from build123d import *

# Parameters (mm, degrees)
SKETCH1_W           = 12.7
SKETCH1_H           = 12.7
BOSS_EXTRUDE1_DEPTH = 2.54
FILLET1_R           = 0.635
SHELL1_START        = 0.635
SHELL1_OUTLINE_W    = 1.905
SHELL1_OUTLINE_H    = 11.43
SHELL1_DEPTH        = 11.43
SKETCH2_R           = 2.54
BOSS_EXTRUDE2_DEPTH = 1.905
BOSS_EXTRUDE3_DEPTH = 0.00254


# Read off the part's stored shape, not the designer's step: Shell1
with BuildPart() as part:
    # Sketch1 → Boss-Extrude1 (new body)
    with BuildSketch(Plane(origin=(0, 0, 0), x_dir=(1, 0, 0), z_dir=(0, 1, 0))):
        with Locations((6.35, 6.35)):
            Rectangle(SKETCH1_W, SKETCH1_H)
    extrude(amount=BOSS_EXTRUDE1_DEPTH)

    # Fillet1
    fillet1_edges = [part.edges().sort_by_distance(p)[0] for p in [
        (0, 1.27, -12.7),
        (12.7, 1.27, -12.7),
        (12.7, 1.27, 0),
        (0, 1.27, 0),
    ]]
    fillet(fillet1_edges, radius=FILLET1_R)

    # Shell1 outline → Shell1 (cut)
    with BuildSketch(Plane.YZ.offset(SHELL1_START)):
        with Locations((0.9525, -6.35)):
            Rectangle(SHELL1_OUTLINE_W, SHELL1_OUTLINE_H)
    extrude(amount=SHELL1_DEPTH, mode=Mode.SUBTRACT)

    # Sketch2 → Boss-Extrude2 (add)
    with BuildSketch(Plane(origin=(0, 1.905, 0), x_dir=(-1, 0, 0), z_dir=(0, -1, 0))):
        with Locations(Location((-6.35, 6.35, 0), (0, 0, 270))):
            Circle(SKETCH2_R)
    extrude(amount=BOSS_EXTRUDE2_DEPTH)

    # Sketch3 → Boss-Extrude3 (add)
    with BuildSketch(Plane(origin=(0, 2.54, 0), x_dir=(1, 0, 0), z_dir=(0, 1, 0))):
        Polygon((4.556857692, 8.001), (5.145173998, 8.001), (5.615191026, 5.974011819), (6.153897957, 8.001), (6.707869311, 8.001), (7.243396154, 5.974011819), (7.712141146, 8.001), (8.301729487, 8.001), (7.567129127, 4.826), (6.971816627, 4.826), (6.42929359, 6.878428886), (5.883590465, 4.826), (5.292730088, 4.826), align=None)
    extrude(amount=BOSS_EXTRUDE3_DEPTH)


solid = part.part
Design review of the part built by this model. Coordinates are the model's own, in mm. A direction names the side the tool comes from. Round coordinates to 2 decimals unless told otherwise and drop trailing zeros. Write each loop counter-clockwise with the first axis right and the second up, starting at its lowest first coordinate (ties: lowest second). Pieces come first, ordered by that corner, then holes. Notation, with made-up numbers: M -15,68.25 L 0,68.25 A13 ccw 0,84.25 Z; hole C 27,89.5 d7. An arc over 180 degrees is marked long. One line per item, written item: value. Start each with the question number.
1. Draft analysis for pull direction Z (two halves, no side actions). For faces 1 (the face through (6, 1, 0)), 2 (the face through (0.635, 1, -6)), 3 (the face through (0, 1, -6)), state which applies: pulls with the +Z half, pulls with the -Z half, needs draft (parallel to the pull), parting line crosses it, or undercut.
2. Take a section at C-C on z = -2.5. State the section outline as (x, y) points (3 decimals), then the cut area to 3 significant figures.
3. Take a section at D-D on z = -8.5. State the section outline as (x, y) points (3 decimals), then the cut area to 3 significant figures.
4. Clearance check with a flat-ended pin moving along its axis: P1, Ø1.5, axis at x = 8, z = -5.5, coming from the +Y side. State where the tip first meets the part, or that it passes through.
5. Take a section at B-B on x = 10.75. State the section outline as (y, z) points (3 decimals).
6. Take a section at A-A on y = 1.7. State the section outline as (x, z) points (3 decimals).
7. To check wall thickness, follow probe 1 along X at (y, z) = (1.5, -6.25) (3 decimals); probe 2 along X at (y, z) = (0.4, -10.25) (3 decimals); probe 3 along Z at (x, y) = (11.5, 0.7) (3 decimals). State the ranges of each line that lie inside material, in increasing order. Write a range as from..to.
8. For faces 4 (the face through (6, 0, -6)), 5 (the face through (5, 1.905, -9)), list the 3-axis set-ups (+Z, -Z, +X, -X, +Y, -Y) from which the entire face can be reached by the end or side of a thin tool; tool diameter is ignored.
Computed:
1. face 1: pulls with the +Z half
1. face 2: undercut
1. face 3: needs draft
2. outline: M 0,0 L 0.635,0 L 0.635,1.905 L 12.065,1.905 L 12.065,0 L 12.7,0 L 12.7,2.54 L 0,2.54 Z
2. area: 10.5 mm²
3. outline: M 0,0 L 0.635,0 L 0.635,1.905 L 4.998,1.905 L 4.998,0 L 7.702,0 L 7.702,1.905 L 12.065,1.905 L 12.065,0 L 12.7,0 L 12.7,2.54 L 0,2.54 Z
3. area: 15.6 mm²
4. P1: stops at y = 2.54
5. outline: M 0,-12.7 L 2.54,-12.7 L 2.54,0 L 0,0 L 0,-0.635 L 1.905,-0.635 L 1.905,-12.065 L 0,-12.065 Z
6. outline: M 0,-12.065 A0.635 ccw 0.635,-12.7 L 12.065,-12.7 A0.635 ccw 12.7,-12.065 L 12.7,-0.635 A0.635 ccw 12.065,0 L 0.635,0 A0.635 ccw 0,-0.635 Z; C 6.35,-6.35 d5.08; hole M 0.635,-12.065 L 12.065,-12.065 L 12.065,-0.635 L 0.635,-0.635 Z
7. probe 1: x = 0..0.635, 3.812..8.888, 12.065..12.7
7. probe 2: x = 0..0.635, 12.065..12.7
7. probe 3: z = -12.7..-12.065, -0.635..0
8. face 4: +Z, -Z, +X, -X, -Y
8. face 5: -Y
